Here's the drawing with two shaded views (mm, measured from the low corner). I have some questions. A direction names the side the tool comes from. Round coordinates to 2 decimals unless told otherwise and drop trailing zeros. Loops run counter-clockwise (first coordinate to the right, second up) from the corner with the lowest first, then second, coordinate; pieces in that order, holes last. Notation, with made-up numbers: (56, -23) -> (103, -23) arc R22 cw to (103, 13) -> close; hole circle Ø6 at (80.5, 51). An arc over 180 degrees is marked (long way). Use a Markdown table: item, result.
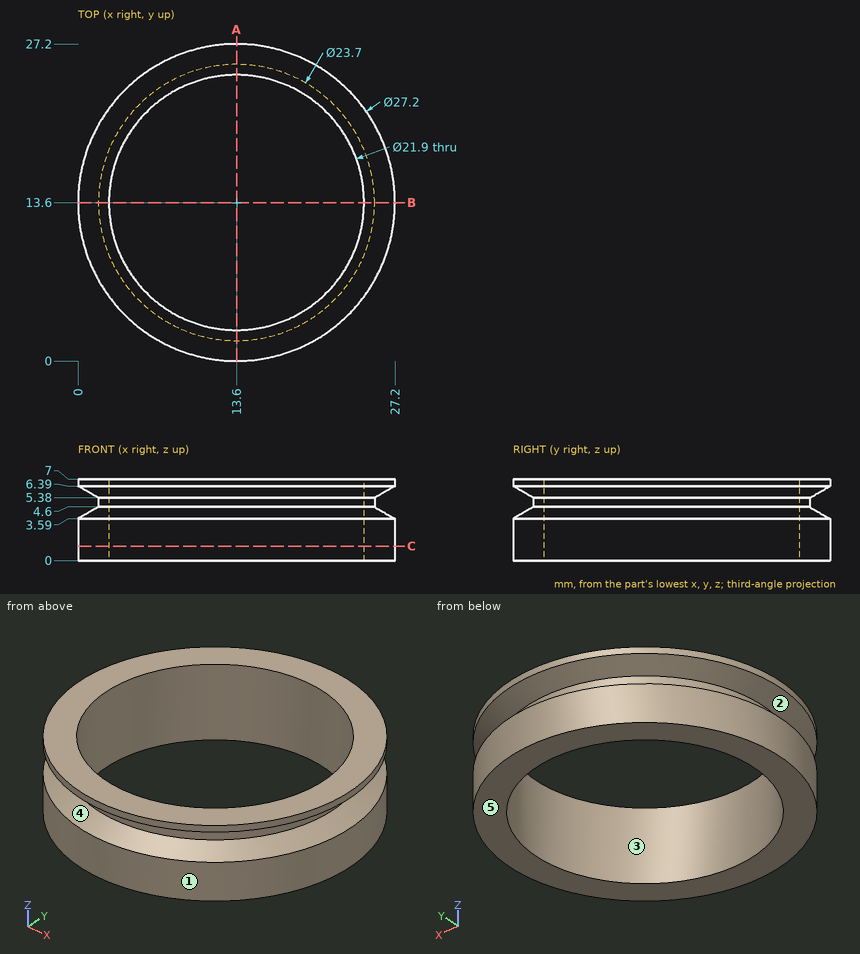
1. I need wall thicknesses on line 1 (Y direction, x = 13.5, z = 2); line 2 (X direction, y = 21.25, z = 4.25) (1 decimal); line 3 (X direction, y = 23.25, z = 1.25) (1 decimal). Which ranges of each line are inside material? Lowest first, please.
Answer sheet:
| item | result |
|---|---|
| line 1 | y = 0 to 2.65, 24.55 to 27.2 |
| line 2 | x = 3.8 to 5.8, 21.4 to 23.4 |
| line 3 | x = 4 to 8.4, 18.8 to 23.2 |
2. Will these pins go through, and if not, where does the flat tip stop? pin 1 Ø1.5 at (y, z) = (22, 1) entering from -X (1 decimal); pin 2 Ø1 at (x, z) = (6.5, 5.5) entering from -Y; pin 3 Ø4 at (y, z) = (5.5, 3) entering from -X (1 decimal).
Answer sheet:
| item | result |
|---|---|
| pin 1 | stops at x = 2.4 |
| pin 2 | stops at y = 2.75 |
| pin 3 | stops at x = 1.4 |
3. I want a section at C-C (z = 1.25). Please give me the cut outline in (x, y), plus the area to 3 significant figures.
Answer sheet:
| item | result |
|---|---|
| outline | circle Ø27.2 at (13.6, 13.6); hole circle Ø21.9 at (13.6, 13.6) |
| area | 204 mm² |
4. Which directions (+Z, -Z, +X, -X, +Y, -Y) give clear straight access to the entire face, cutting with the end or side of a thin tool? Please do the marked faces 1 and 2.
Answer sheet:
| item | result |
|---|---|
| face 1 | +Z, -Z |
| face 2 | none |
5. If we mould it in two halves opening along X, with no side actions, what happens to the marked faces 3, 4 and 5? For each: +X half, -X half, draft (parallel to the pull), parting line (faces both ways), or undercut.
Answer sheet:
| item | result |
|---|---|
| face 3 | undercut |
| face 4 | parting line |
| face 5 | draft |
6. I want a section at A-A (x = 13.6). Please give me the cut outline in (y, z).
Answer sheet:
| item | result |
|---|---|
| outline | (0, 0) -> (2.65, 0) -> (2.65, 7) -> (0, 7) -> (0, 6.39) -> (1.75, 5.38) -> (1.75, 4.6) -> (0, 3.59) -> close; (24.55, 0) -> (27.2, 0) -> (27.2, 3.59) -> (25.45, 4.6) -> (25.45, 5.38) -> (27.2, 6.39) -> (27.2, 7) -> (24.55, 7) -> close |
